```python
from build123d import *

# Parameters (mm, degrees)
F0_R          = 10
F0_R_2        = 5
F1_DEPTH      = 7
F2_SIZE       = 1
F3_R          = 11.3100370754
F4_DEPTH      = 25
F4_DEPTH_BACK = 25


with BuildPart() as f1:
    # F0 (on Top) → F1 (new body)
    with BuildSketch(Plane.XY):
        Circle(F0_R)
        Circle(F0_R_2, mode=Mode.SUBTRACT)
    extrude(amount=F1_DEPTH)

    # F2
    f2_edges = [f1.edges().sort_by_distance(p)[0] for p in [
        (-10, 0, 7),
        (-10, 0, 0),
    ]]
    chamfer(f2_edges, length=F2_SIZE)

    # F3 (on Top) → F4 (cut, two sides)
    with BuildSketch(Plane.XY) as f4_sk:
        Circle(F3_R)
        Polygon((-0.8305830461, 10.0236467025), (0, 9.4011723995), (0.8305830461, 10.0236467025), (1.5473821193, 9.2729526615), (2.4690929981, 9.7502277502), (3.052555688, 8.8917909477), (4.0402525295, 9.2108480018), (4.474463495, 8.2680843559), (5.5012045041, 8.4202203307), (5.774319602, 7.4188459763), (6.8120979603, 7.399910999), (6.9166673227, 6.3672408179), (7.937175142, 6.1777513853), (7.8703463892, 5.1419539281), (8.8457468766, 4.787078818), (8.6093429228, 3.7764079393), (9.5130296954, 3.2658272195), (9.1134990242, 2.3078513862), (9.9208218628, 1.6554923679), (9.3690626294, 0.7763426634), (10.0579998714, 0), (9.3690626294, -0.7763426634), (9.9208218628, -1.6554923679), (9.1134990242, -2.3078513862), (9.5130296954, -3.2658272195), (8.6093429228, -3.7764079393), (8.8457468766, -4.787078818), (7.8703463892, -5.1419539281), (7.937175142, -6.1777513853), (6.9166673227, -6.3672408179), (6.8120979603, -7.399910999), (5.774319602, -7.4188459763), (5.5012045041, -8.4202203307), (4.474463495, -8.2680843559), (4.0402525295, -9.2108480018), (3.052555688, -8.8917909477), (2.4690929981, -9.7502277502), (1.5473821193, -9.2729526615), (0.8305830461, -10.0236467025), (0, -9.4011723995), (-0.8305830461, -10.0236467025), (-1.5473821193, -9.2729526615), (-2.4690929981, -9.7502277502), (-3.052555688, -8.8917909477), (-4.0402525295, -9.2108480018), (-4.474463495, -8.2680843559), (-5.5012045041, -8.4202203307), (-5.774319602, -7.4188459763), (-6.8120979603, -7.399910999), (-6.9166673227, -6.3672408179), (-7.937175142, -6.1777513853), (-7.8703463892, -5.1419539281), (-8.8457468766, -4.787078818), (-8.6093429228, -3.7764079393), (-9.5130296954, -3.2658272195), (-9.1134990242, -2.3078513862), (-9.9208218628, -1.6554923679), (-9.3690626294, -0.7763426634), (-10.0579998714, 0), (-9.3690626294, 0.7763426634), (-9.9208218628, 1.6554923679), (-9.1134990242, 2.3078513862), (-9.5130296954, 3.2658272195), (-8.6093429228, 3.7764079393), (-8.8457468766, 4.787078818), (-7.8703463892, 5.1419539281), (-7.937175142, 6.1777513853), (-6.9166673227, 6.3672408179), (-6.8120979603, 7.399910999), (-5.774319602, 7.4188459763), (-5.5012045041, 8.4202203307), (-4.474463495, 8.2680843559), (-4.0402525295, 9.2108480018), (-3.052555688, 8.8917909477), (-2.4690929981, 9.7502277502), (-1.5473821193, 9.2729526615), align=None, mode=Mode.SUBTRACT)
    extrude(amount=-F4_DEPTH, mode=Mode.SUBTRACT)
    extrude(f4_sk.sketch, amount=F4_DEPTH_BACK, mode=Mode.SUBTRACT)


solid = f1.part
```
For this review, take the finished solid that the model builds, in its own axes (mm). A direction names the side the tool comes from. Round coordinates to 2 decimals unless told otherwise and drop trailing zeros. One line per item, written item: value. Start each with the question number.
(1) Wall thickness on line 1 (Y direction, x = -4.25, z = 3.25); line 2 (Y direction, x = 2, z = 6); line 3 (X direction, y = 2, z = 3.25): over which ranges is each line inside the solid? List them lowest first.
(2) Machinability: for faces 5 (the flat face through (-4.938, -8.337, 3.457)), 6 (the flat face through (9.03, -3.54, 3.46)), 7 (the flat face through (-9.017, -3.546, 3.457)), 8 (the flat face through (4.938, 8.337, 3.457)), 9 (the conical face through (8.74, 2.75, 6.84)), which of the approach directions +Z, -Z, +X, -X, +Y, -Y give a long, thin tool a straight path to every point of the face, cutting with its end or side? Answer none if there is none.
(3) Insertion check: pin 1 (4 mm diameter, centred on y = 5.5, z = 6, fed in from -X); pin 2 (3 mm diameter, centred on x = 2.5, z = 6.5, fed in from +Y); pin 3 (1 mm diameter, centred on y = 5, z = 2, fed in from +X). Each pin has a flat end and moves straight along its axis. Give the tip position at first contact, or say it passes through.
(4) The part is to be moulded in two halves that separate along Y. For faces 1 (the flat face through (-8.716, 4.233, 3.457)), 2 (the flat face through (7.9, -5.6, 3.5)), 3 (the flat face through (5.65, 7.88, 3.46)), 4 (the flat face through (6.87, -6.83, 3.46)), say which applies: released by +Y, released by -Y, zero draft, split by the parting line, or undercut.
Result:
1. line 1: -8.76 to -2.63, 2.63 to 8.76
1. line 2: -9.51 to -4.58, 4.58 to 9.51
1. line 3: -9.49 to -4.58, 4.58 to 9.49
2. face 5: +Z, -Z, -Y
2. face 6: +Z, -Z, +X
2. face 7: +Z, -Z, -X
2. face 8: +Z, -Z, +Y
2. face 9: +Z
3. pin 1: x = -9.1
3. pin 2: y = 9.8
3. pin 3: x = 8.83
4. face 1: undercut
4. face 2: undercut
4. face 3: released by +Y
4. face 4: released by -Y
